```python
from build123d import *

# Parameters (mm, degrees)
SKETCH1_W           = 52
SKETCH1_H           = 200
BOSS_EXTRUDE1_DEPTH = 6
SKETCH2_R           = 1.5
CUT_EXTRUDE2_DEPTH  = 6
SKETCH3_R           = 1.5
CUT_EXTRUDE4_DEPTH  = 6
SKETCH4_R           = 1.5
CUT_EXTRUDE6_DEPTH  = 6
SKETCH5_R           = 1.5
CUT_EXTRUDE8_DEPTH  = 6
SKETCH6_R           = 1.5
CUT_EXTRUDE10_DEPTH = 6
SKETCH7_R           = 1.5
CUT_EXTRUDE12_DEPTH = 6
SKETCH8_R           = 1.5
CUT_EXTRUDE14_DEPTH = 6
SKETCH9_R           = 1.5
CUT_EXTRUDE16_DEPTH = 6
SKETCH10_R          = 1.5
CUT_EXTRUDE18_DEPTH = 6
SKETCH11_R          = 1.5
CUT_EXTRUDE20_DEPTH = 6
SKETCH12_R          = 1.5
CUT_EXTRUDE22_DEPTH = 6
SKETCH13_R          = 1.5
CUT_EXTRUDE24_DEPTH = 6
SKETCH14_W          = 36
SKETCH14_H          = 37
CUT_EXTRUDE26_DEPTH = 6
SKETCH15_W          = 36
SKETCH15_H          = 37
CUT_EXTRUDE28_DEPTH = 6


with BuildPart() as part:
    # Sketch1 → Boss-Extrude1 (new body)
    with BuildSketch(Plane(origin=(-132.7, 0, 0), x_dir=(0, 0, -1), z_dir=(1, 0, 0))):
        Rectangle(SKETCH1_W, SKETCH1_H)
    extrude(amount=BOSS_EXTRUDE1_DEPTH)

    # Sketch2 → Cut-Extrude2 (cut)
    with BuildSketch(Plane(origin=(-132.7, 0, 0), x_dir=(0, 0, -1), z_dir=(1, 0, 0))):
        with Locations((-4, 84)):
            Circle(SKETCH2_R)
    extrude(amount=CUT_EXTRUDE2_DEPTH, mode=Mode.SUBTRACT)

    # Sketch3 → Cut-Extrude4 (cut)
    with BuildSketch(Plane(origin=(-132.7, 0, 0), x_dir=(0, 0, -1), z_dir=(1, 0, 0))):
        with Locations((4, 84)):
            Circle(SKETCH3_R)
    extrude(amount=CUT_EXTRUDE4_DEPTH, mode=Mode.SUBTRACT)

    # Sketch4 → Cut-Extrude6 (cut)
    with BuildSketch(Plane(origin=(-132.7, 0, 0), x_dir=(0, 0, -1), z_dir=(1, 0, 0))):
        with Locations((-4, 92)):
            Circle(SKETCH4_R)
    extrude(amount=CUT_EXTRUDE6_DEPTH, mode=Mode.SUBTRACT)

    # Sketch5 → Cut-Extrude8 (cut)
    with BuildSketch(Plane(origin=(-132.7, 0, 0), x_dir=(0, 0, -1), z_dir=(1, 0, 0))):
        with Locations((4, 92)):
            Circle(SKETCH5_R)
    extrude(amount=CUT_EXTRUDE8_DEPTH, mode=Mode.SUBTRACT)

    # Sketch6 → Cut-Extrude10 (cut)
    with BuildSketch(Plane(origin=(-132.7, 0, 0), x_dir=(0, 0, -1), z_dir=(1, 0, 0))):
        with Locations((-4, -92)):
            Circle(SKETCH6_R)
    extrude(amount=CUT_EXTRUDE10_DEPTH, mode=Mode.SUBTRACT)

    # Sketch7 → Cut-Extrude12 (cut)
    with BuildSketch(Plane(origin=(-132.7, 0, 0), x_dir=(0, 0, -1), z_dir=(1, 0, 0))):
        with Locations((4, -92)):
            Circle(SKETCH7_R)
    extrude(amount=CUT_EXTRUDE12_DEPTH, mode=Mode.SUBTRACT)

    # Sketch8 → Cut-Extrude14 (cut)
    with BuildSketch(Plane(origin=(-132.7, 0, 0), x_dir=(0, 0, -1), z_dir=(1, 0, 0))):
        with Locations((-4, -84)):
            Circle(SKETCH8_R)
    extrude(amount=CUT_EXTRUDE14_DEPTH, mode=Mode.SUBTRACT)

    # Sketch9 → Cut-Extrude16 (cut)
    with BuildSketch(Plane(origin=(-132.7, 0, 0), x_dir=(0, 0, -1), z_dir=(1, 0, 0))):
        with Locations((4, -84)):
            Circle(SKETCH9_R)
    extrude(amount=CUT_EXTRUDE16_DEPTH, mode=Mode.SUBTRACT)

    # Sketch10 → Cut-Extrude18 (cut)
    with BuildSketch(Plane(origin=(-132.7, 0, 0), x_dir=(0, 0, -1), z_dir=(1, 0, 0))):
        with Locations((-15, -30)):
            Circle(SKETCH10_R)
    extrude(amount=CUT_EXTRUDE18_DEPTH, mode=Mode.SUBTRACT)

    # Sketch11 → Cut-Extrude20 (cut)
    with BuildSketch(Plane(origin=(-132.7, 0, 0), x_dir=(0, 0, -1), z_dir=(1, 0, 0))):
        with Locations((15, -30)):
            Circle(SKETCH11_R)
    extrude(amount=CUT_EXTRUDE20_DEPTH, mode=Mode.SUBTRACT)

    # Sketch12 → Cut-Extrude22 (cut)
    with BuildSketch(Plane(origin=(-132.7, 0, 0), x_dir=(0, 0, -1), z_dir=(1, 0, 0))):
        with Locations((-15, 30)):
            Circle(SKETCH12_R)
    extrude(amount=CUT_EXTRUDE22_DEPTH, mode=Mode.SUBTRACT)

    # Sketch13 → Cut-Extrude24 (cut)
    with BuildSketch(Plane(origin=(-132.7, 0, 0), x_dir=(0, 0, -1), z_dir=(1, 0, 0))):
        with Locations((15, 30)):
            Circle(SKETCH13_R)
    extrude(amount=CUT_EXTRUDE24_DEPTH, mode=Mode.SUBTRACT)

    # Sketch14 → Cut-Extrude26 (cut)
    with BuildSketch(Plane(origin=(-132.7, 0, 0), x_dir=(0, 0, -1), z_dir=(1, 0, 0))):
        with Locations((0, 53.5)):
            Rectangle(SKETCH14_W, SKETCH14_H)
    extrude(amount=CUT_EXTRUDE26_DEPTH, mode=Mode.SUBTRACT)

    # Sketch15 → Cut-Extrude28 (cut)
    with BuildSketch(Plane(origin=(-132.7, 0, 0), x_dir=(0, 0, -1), z_dir=(1, 0, 0))):
        with Locations((0, -53.5)):
            Rectangle(SKETCH15_W, SKETCH15_H)
    extrude(amount=CUT_EXTRUDE28_DEPTH, mode=Mode.SUBTRACT)


solid = part.part
```
CAD build for the part. Positions are in the model's coordinates, mm. A direction names the side the tool comes from. Round coordinates to 2 decimals unless told otherwise and drop trailing zeros. Answer in a Markdown table with one row per item. Add a question column.
Item 1: Drill centre lines: line 1 (Z direction, x = -128.8, y = 92); line 2 (Y direction, x = -129.15, z = 1.5); line 3 (Y direction, x = -129.7, z = -15). Where is each one in solid material? Low to high. Write a range as from..to.
Item 2: Mould opens along Y. For faces 1 (the face through (-130, -1, 26)), 2 (the face through (-130, -100, 0)), 3 (the face through (-130, -35, 0)) say: pulls with the +Y half, pulls with the -Y half, needs draft (parallel to the pull), parting line crosses it, or undercut.
Item 3: Which spindle directions (+Z, -Z, +X, -X, +Y, -Y) get a long thin tool onto all of the face, cutting with end or side? Do faces 4 (the face through (-130, -1, -26)), 5 (the face through (-130, 35, 0)). Say none if no direction does.
Item 4: Saw through at A-A, the plane x = -128.2. Count the separate pieces of the cut face and the enclosed holes in it, then the cut area to 3 significant figures.
Item 5: Drop flat-ended pins along their axis: pin 1 Ø2.5 at (y, z) = (-92, 4) entering from +X; pin 2 Ø3.5 at (y, z) = (30, -15) entering from +X. Give the stop position or say it passes through.
Findings below:
| question | item | result |
|---|---|---|
| 1 | line 1 | z = -26..-5.5, -2.5..2.5, 5.5..26 |
| 1 | line 2 | y = -100..-72, -35..35, 72..100 |
| 1 | line 3 | y = -100..-72, -35..-31.5, -28.5..28.5, 31.5..35, 72..100 |
| 2 | face 1 | needs draft |
| 2 | face 2 | pulls with the -Y half |
| 2 | face 3 | undercut |
| 3 | face 4 | -Z, +X, -X, +Y, -Y |
| 3 | face 5 | +X, -X |
| 4 | separate pieces | 1 |
| 4 | enclosed holes | 14 |
| 4 | area | 7,650 mm^2 |
| 5 | pin 1 | passes through |
| 5 | pin 2 | stops at x = -126.7 |
